```python
from build123d import *

# Parameters (mm, degrees)
SKETCH_2_W      = 1.5
SKETCH_2_H      = 5
EXTRUDE_1_DEPTH = 10


with BuildPart() as part:
    # Эскиз1 → Повернуть1 (revolve)
    with BuildSketch(Plane.XY, mode=Mode.PRIVATE) as revolve_1_sk:
        Polygon((0, 0), (0, 18.5), (57, 18.5), (57, 26), (95, 26), (95, 28.5), (121, 22.5), (121, 6), (124, 6), (124, 20), (164, 20), (176, 8), (176, 5), (166, 5), (166, 0), align=None)
    revolve(revolve_1_sk.sketch.rotate(Axis((0, 0, 0), (1, 0, 0)), 90), axis=Axis((0, 0, 0), (1, 0, 0)))

    # Эскиз2 → Бобышка-Вытянуть1 (add)
    with BuildSketch(Plane.ZY):
        with Locations((10.556652869, 0)):
            Rectangle(SKETCH_2_W, SKETCH_2_H)
        with Locations((-10.556652869, 0)):
            Rectangle(SKETCH_2_W, SKETCH_2_H)
    extrude(amount=EXTRUDE_1_DEPTH)


solid = part.part
```
Work out the finished part from the listing and answer in its coordinate system (mm). A direction names the side the tool comes from. Coordinates: 2 decimals unless noted, no trailing zeros. Write each loop counter-clockwise with the first axis right and the second up, starting at its lowest first coordinate (ties: lowest second). Pieces come first, ordered by that corner, then holes. Notation, with made-up numbers: (82, 64) - (93, 64) arc R18 cw to (93, 80) - close; hole circle Ø4 at (54, 23.5). An arc over 180 degrees is marked (long way). Answer as a JSON object with one key per item and string values.
Q1. Find section D-D (x = 116.5). Write down the section's boundary in (y, z).
Results list:
{"outline": "circle Ø47.08 at (0, 0)"}
Q2. For a pull along Z with two mould halves and no side action, classify faces 1 (the flat face through (-5, 0, -11.307)), 2 (the cylindrical face through (122.521, -1.802, 5.723)), 3 (the flat face through (-5, 0, -9.807)) as pulls with the +Z half, pulls with the -Z half, needs draft (parallel to the pull), parting line crosses it, or undercut.
Results list:
{"face 1": "pulls with the -Z half", "face 2": "parting line crosses it", "face 3": "undercut"}
Q3. Given pin 1 Ø1.5 at (x, y) = (86.5, 1.5) entering from +Z; pin 2 Ø3 at (y, z) = (1.5, -1) entering from +X; pin 3 Ø12 at (y, z) = (9.5, 20.5) entering from +X, each flat-ended and moving along its own axis, determine where each tip first touches the part or whether it passes through.
Results list:
{"pin 1": "stops at z = 25.99", "pin 2": "stops at x = 166", "pin 3": "stops at x = 167.41"}
Q4. Which of the six approach directions +Z, -Z, +X, -X, +Y, -Y give full straight-line access (tool end or side, diameter ignored) to faces 4 (the flat face through (124, -5, -4)), 5 (the cylindrical face through (76.266, 15.821, -20.633)), 6 (the cylindrical face through (144.28, -0.88, -19.98))?
Results list:
{"face 4": "none", "face 5": "-X", "face 6": "+X"}
Q5. Consider L1, parallel to X at y = -4.5, z = -11; L2, parallel to X at y = 16.5, z = 14.5; L3, parallel to Y at x = 173.25, z = 0. Determine where each line is inside the solid, lowest interval first. Write a range as from..to.
Results list:
{"L1": "x = 0..121, 124..172.12", "L2": "x = 57..121", "L3": "y = -10.75..-5, 5..10.75"}
Q6. Find section A-A (z = 0). Write down the section's boundary in (x, y), plus the area to 3 significant figures.
Results list:
{"outline": "(0, -18.5) - (57, -18.5) - (57, -26) - (95, -26) - (95, -28.5) - (121, -22.5) - (121, -6) - (124, -6) - (124, -20) - (164, -20) - (176, -8) - (176, -5) - (166, -5) - (166, 5) - (176, 5) - (176, 8) - (164, 20) - (124, 20) - (124, 6) - (121, 6) - (121, 22.5) - (95, 28.5) - (95, 26) - (57, 26) - (57, 18.5) - (0, 18.5) - close", "area": "7,280 mm^2"}
Q7. Find section C-C (x = 68). Write down the section's boundary in (y, z).
Results list:
{"outline": "circle Ø52 at (0, 0)"}
